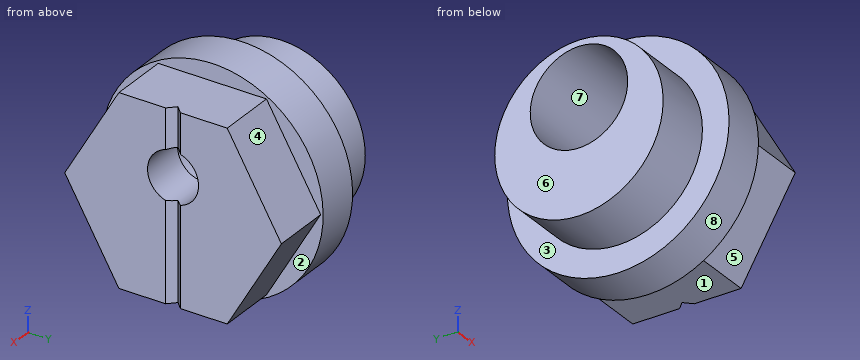
```python
from build123d import *

# Parameters (mm, degrees)
SKETCH1_W                                      = 3
SKETCH1_H                                      = 7.5
BOSS_EXTRUDE1_DEPTH                            = 4
CUT_EXTRUDE1_DEPTH                             = 14.85
SKETCH4_R                                      = 5.7
BOSS_EXTRUDE2_DEPTH                            = 4
CBORE_FOR_5_BUTTON_HEAD_CAP_SCREW1_D           = 1.5875
CBORE_FOR_5_BUTTON_HEAD_CAP_SCREW1_CBORE_D     = 6.600000008
CBORE_FOR_5_BUTTON_HEAD_CAP_SCREW1_CBORE_DEPTH = 7.9375
F_8_32_TAPPED_HOLE1_D                          = 3.4544


with BuildPart() as part:
    # Sketch1 → Revolve1 (revolve)
    with BuildSketch(Plane.XY, mode=Mode.PRIVATE) as revolve1_sk:
        with Locations((5.5, 3.75)):
            Rectangle(SKETCH1_W, SKETCH1_H)
    revolve(revolve1_sk.sketch.rotate(Axis((4, 0, 0), (1, 0, 0)), 270), axis=Axis((4, 0, 0), (1, 0, 0)))  # turned: the seam where the file's is

    # Sketch2 → Boss-Extrude1 (add)
    with BuildSketch(Plane(origin=(7, 0, 0), x_dir=(0, 0, -1), z_dir=(1, 0, 0))):
        Polygon((0, -7.332348419), (-6.35, -3.666174209), (-6.35, 3.666174209), (0, 7.332348419), (6.35, 3.666174209), (6.35, -3.666174209), align=None)
    extrude(amount=BOSS_EXTRUDE1_DEPTH)

    # Sketch3 → Cut-Extrude1 (cut, through all)
    with BuildSketch(Plane.XY.offset(6.35)):
        Polygon((11, -0.5), (11, 0.5), (10.5, 0), align=None)
    extrude(amount=-CUT_EXTRUDE1_DEPTH, mode=Mode.SUBTRACT)

    # Sketch4 → Boss-Extrude2 (add)
    with BuildSketch(Plane.ZY.offset(-4)):
        Circle(SKETCH4_R)
    extrude(amount=BOSS_EXTRUDE2_DEPTH)

    # CBORE for #5 Button Head Cap Screw1 (through all)
    with Locations(Plane.ZY):
        with Locations((2, 0)):
            CounterBoreHole(CBORE_FOR_5_BUTTON_HEAD_CAP_SCREW1_D / 2, CBORE_FOR_5_BUTTON_HEAD_CAP_SCREW1_CBORE_D / 2, CBORE_FOR_5_BUTTON_HEAD_CAP_SCREW1_CBORE_DEPTH)

    # #8-32 Tapped Hole1 (through all)
    with Locations(Plane(origin=(11, 0, 0), x_dir=(0, 0, -1), z_dir=(1, 0, 0))):
        with Locations((-2, 0)):
            Hole(F_8_32_TAPPED_HOLE1_D / 2)


solid = part.part
```
CAD build for the part. Positions are in the model's coordinates, mm. Face numbers are marked on the shaded views. A direction names the side the tool comes from. Coordinates: 2 decimals unless noted, no trailing zeros. Order: outer loops, then holes, each group sorted by start corner. A loop starts at its lowest first (then second) coordinate and runs counter-clockwise, first axis right, second up. Notation, with made-up numbers: (36, -13) -> (68, -13) arc R23 ccw to (68, 2) -> close; hole circle Ø7 at (-20, 13.25). An arc over 180 degrees is marked (long way). Use one line per item in the form item = value. Start each with the question number.
1) Band-saw the part on C-C on y = 5.25. Give the cut face in (x, z), then the cut area to 3 significant figures.
2) Pull direction Y, two halves, no side cores. Call the marked faces 6, 7 and 8: +Y half, -Y half, draft (parallel to the pull), parting line (faces both ways), or undercut.
3) Tool access for the marked faces 1, 2, 3, 4 and 5: list every direction of +Z, -Z, +X, -X, +Y, -Y with a clear straight run to the whole face (end or side of a thin tool).
4) Drill centre lines: L1, parallel to Z at x = 10.15, y = 0; L2, parallel to X at y = 3.25, z = 1.75; L3, parallel to X at y = 0.25, z = -6.5. Where is each one in solid material? Low to high. Write a range as [from, to].
5) Band-saw the part on D-D on x = 4.5. Give the cut face in (y, z).
6) Drop flat-ended pins along their axis: pin 1 (2 mm diameter, centred on x = 9.5, y = -1, fed in from -Z); pin 2 (1.5 mm diameter, centred on x = 3, z = -4, fed in from -Y); pin 3 (1 mm diameter, centred on x = 5.5, z = 2, fed in from -Y); pin 4 (2 mm diameter, centred on y = 0, z = 2, fed in from -X). Give the stop position or say it passes through.
7) Band-saw the part on B-B on x = 7.5. Give the cut face in (y, z).
8) Band-saw the part on A-A on z = 2. Give the cut face in (x, y), then the cut area to 3 significant figures.
Entries:
q1.outline = (0, -2.22) -> (4, -2.22) -> (4, -5.36) -> (7, -5.36) -> (7, -3.61) -> (11, -3.61) -> (11, 3.61) -> (7, 3.61) -> (7, 5.36) -> (4, 5.36) -> (4, 2.22) -> (0, 2.22) -> close
q1.area = 78.7 mm2
q2.face_6 = draft
q2.face_7 = undercut
q2.face_8 = parting line
q3.face_1 = -Z, +X, +Y, -Y
q3.face_2 = +X
q3.face_3 = -X
q3.face_4 = +Z, +X, +Y
q3.face_5 = -Z, +X, -Y
q4.L1 = [-6.35, 0.27], [3.73, 6.35]
q4.L2 = [7.94, 11]
q4.L3 = [4, 7]
q5.outline = circle Ø15 at (0, 0); hole circle Ø6.6 at (0, 2)
q6.pin_1 = -6.35
q6.pin_2 = -4.68
q6.pin_3 = -7.35
q6.pin_4 = through
q7.outline = (-7.33, 0) -> (-3.67, -6.35) -> (3.67, -6.35) -> (7.33, 0) -> (3.67, 6.35) -> (-3.67, 6.35) -> close; hole circle Ø6.6 at (0, 2)
q8.outline = (0, -5.34) -> (4, -5.34) -> (4, -7.23) -> (7, -7.23) -> (7, -6.18) -> (11, -6.18) -> (11, -1.73) -> (7.94, -1.73) -> (7.94, -3.3) -> (0, -3.3) -> close; (0, 3.3) -> (7.94, 3.3) -> (7.94, 1.73) -> (11, 1.73) -> (11, 6.18) -> (7, 6.18) -> (7, 7.23) -> (4, 7.23) -> (4, 5.34) -> (0, 5.34) -> close
q8.area = 72.5 mm2
